```python
from build123d import *

# Parameters (mm, degrees)
SKETCH_1_R          = 1.5
SKETCH_1_W          = 1.5
SKETCH_1_H          = 40
EXTRUDE_1_DEPTH     = 1.5
CUT_EXTRUDE_2_DEPTH = 51.351266121
FILLET_1_R          = 4


with BuildPart() as part:
    # 草图1 → 凸台-拉伸1 (new body)
    with BuildSketch(Plane(origin=(0, 0, 0), x_dir=(1, 0, 0), z_dir=(0, 1, 0))):
        Polygon((-33, 25), (-33, -25), (25, -38), (25, 38), align=None)
        with Locations(Location((-25, 16, 0), (0, 0, 270))):
            Circle(SKETCH_1_R, mode=Mode.SUBTRACT)
        with Locations(Location((20, 31, 0), (0, 0, 270))):
            Circle(SKETCH_1_R, mode=Mode.SUBTRACT)
        with Locations(Location((20, -31, 0), (0, 0, 90))):
            Circle(SKETCH_1_R, mode=Mode.SUBTRACT)
        with Locations(Location((-25, -16, 0), (0, 0, 90))):
            Circle(SKETCH_1_R, mode=Mode.SUBTRACT)
        with Locations((-29, 0)):
            Rectangle(SKETCH_1_W, SKETCH_1_H, mode=Mode.SUBTRACT)
    extrude(amount=EXTRUDE_1_DEPTH)

    # 草图3 → 切除-拉伸2 (cut, through all)
    with BuildSketch(Plane(origin=(0, 1.5, 0), x_dir=(1, 0, 0), z_dir=(0, 1, 0))):
        with BuildLine():
            Line((20, -15), (20, 15))
            ThreePointArc((20, 15), (25, 20), (30, 15))
            Line((30, 15), (30, -15))
            ThreePointArc((30, -15), (25, -20), (20, -15))
        make_face()
    extrude(amount=-CUT_EXTRUDE_2_DEPTH, mode=Mode.SUBTRACT)

    # 圆角1
    fillet_1_edges = [part.edges().sort_by_distance(p)[0] for p in [
        (25, 0.75, -38),
        (25, 0.75, 38),
        (-33, 0.75, 25),
        (-33, 0.75, -25),
    ]]
    fillet(fillet_1_edges, radius=FILLET_1_R)


solid = part.part
```
Design review of the part built by this model. Coordinates are the model's own, in mm. A direction names the side the tool comes from. Give positions to 0.01 mm unless a question says otherwise; leave off trailing zeros. Loops run counter-clockwise (first coordinate to the right, second up) from the corner with the lowest first, then second, coordinate; pieces in that order, holes last. Notation, with made-up numbers: (29.25, 57.25) -> (35.25, 57.25) arc R5 ccw to (35.25, 66.25) -> close; hole circle Ø2 at (4, -31). An arc over 180 degrees is marked (long way). Write each question's results on one line, items separated by ' | '.
Q1. Wall thickness on L1, parallel to Z at x = 19.5, y = 0.7; L2, parallel to X at y = 0.6, z = -16; L3, parallel to X at y = 0.2, z = -1: over which ranges is each line inside the solid? List them lowest first.
Reply:
L1: z = -36.77 to -32.41, -29.59 to 29.59, 32.41 to 36.77 | L2: x = -33 to -29.75, -28.25 to -26.5, -23.5 to 20.1 | L3: x = -33 to -29.75, -28.25 to 20
Q2. Take a section at A-A, the plane z = 0.5. Write out the cut boundary in (x, y), plus the area to 4 significant figures.
Reply:
outline: (-33, 0) -> (-29.75, 0) -> (-29.75, 1.5) -> (-33, 1.5) -> close; (-28.25, 0) -> (20, 0) -> (20, 1.5) -> (-28.25, 1.5) -> close | area: 77.25 mm²
Q3. For pin 1 Ø0.8 at (y, z) = (1, 4.5) entering from +X, flat-tipped, find the tip position at first contact; note if it passes through.
Reply:
pin 1: stops at x = 20
Q4. Take a section at D-D, the plane z = -16. Write out the cut boundary in (x, y).
Reply:
outline: (-33, 0) -> (-29.75, 0) -> (-29.75, 1.5) -> (-33, 1.5) -> close; (-28.25, 0) -> (-26.5, 0) -> (-26.5, 1.5) -> (-28.25, 1.5) -> close; (-23.5, 0) -> (20.1, 0) -> (20.1, 1.5) -> (-23.5, 1.5) -> close
Q5. Take a section at B-B, the plane y = 1.05. Write out the cut boundary in (x, z).
Reply:
outline: (-33, -21.8) arc R4 ccw to (-29.87, -25.7) -> (20.13, -36.91) arc R4 ccw to (25, -33) -> (25, -20) arc R5 cw to (20, -15) -> (20, 15) arc R5 cw to (25, 20) -> (25, 33) arc R4 ccw to (20.13, 36.91) -> (-29.87, 25.7) arc R4 ccw to (-33, 21.8) -> close; hole (-29.75, -20) -> (-28.25, -20) -> (-28.25, 20) -> (-29.75, 20) -> close; hole circle Ø3 at (-25, -16); hole circle Ø3 at (-25, 16); hole circle Ø3 at (20, -31); hole circle Ø3 at (20, 31)
Q6. The part is to be moulded in two halves that separate along X. For faces 4 (the face through (20, 1, 0)), 5 (the face through (-4, 0, -1)), 6 (the face through (-32.146, 0.76, 24.268)), 7 (the face through (18.99, 0.74, 32.11)), say which applies: +X half, -X half, draft (parallel to the pull), parting line (faces both ways), or undercut.
Reply:
face 4: +X half | face 5: draft | face 6: -X half | face 7: undercut
Q7. Machinability: for faces 1 (the face through (22, 1, 19)), 2 (the face through (-4, 1.5, -1)), 3 (the face through (-29, 1, 20)), which of the approach directions +Z, -Z, +X, -X, +Y, -Y give a long, thin tool a straight path to every point of the face, cutting with its end or side? Answer none if there is none.
Reply:
face 1: +X, +Y, -Y | face 2: +Z, -Z, +X, -X, +Y | face 3: +Y, -Y
Q8. Take a section at C-C, the plane x = -25. Write out the cut boundary in (y, z).
Reply:
outline: (0, -26.79) -> (1.5, -26.79) -> (1.5, -17.5) -> (0, -17.5) -> close; (0, -14.5) -> (1.5, -14.5) -> (1.5, 14.5) -> (0, 14.5) -> close; (0, 17.5) -> (1.5, 17.5) -> (1.5, 26.79) -> (0, 26.79) -> close
